Build history of the part. All positions in model axes, mm. Face numbers are marked on the shaded views. A direction names the side the tool comes from. Round coordinates to 2 decimals unless told otherwise and drop trailing zeros. Write each loop counter-clockwise with the first axis right and the second up, starting at its lowest first coordinate (ties: lowest second). Pieces come first, ordered by that corner, then holes. Notation, with made-up numbers: (45.25, 75) - (52.25, 75) arc R24 ccw to (52.25, 89) - close; hole circle Ø10 at (70, 66.25). An arc over 180 degrees is marked (long way). Answer as a JSON object with one key per item and string values. Group by question number.
Item 1: Two-plate mould, pull along Y, no slides. Class the marked faces 4, 5 and 6: +Y half, -Y half, draft (parallel to the pull), parting line (faces both ways), or undercut.
Item 2: Which spindle directions (+Z, -Z, +X, -X, +Y, -Y) get a long thin tool onto all of the face, cutting with end or side? Do the marked faces 1, 2 and 3. Say none if no direction does.
Item 3: Slice it at A-A, the plane x = 0. List the corners of the cut face in (y, z).
Item 4: Probe line 1 (Y direction, x = -15.5, z = 30.25); line 2 (X direction, y = -15.5, z = 0.7); line 3 (Y direction, x = 0, z = 33.45). List the from-to ranges inside material, lowest first. Write a range as from..to.
Item 5: Slice it at B-B, the plane z = 4. List the corners of the cut face in (x, y).
Item 6: Flat gauge pins, fed straight in: pin 1 (1.5 mm diameter, centred on y = 14, z = 35, fed in from -X); pin 2 (2 mm diameter, centred on x = -16.5, y = -11, fed in from +Z); pin 3 (0.9 mm diameter, centred on x = -16, y = -15.5, fed in from +Z); pin 4 (5 mm diameter, centred on x = 15.5, y = 15.5, fed in from -Z). Where does each tip first touch, or does it go through?
Item 7: Slice it at D-D, the plane z = 20. List the corners of the cut face in (x, y).
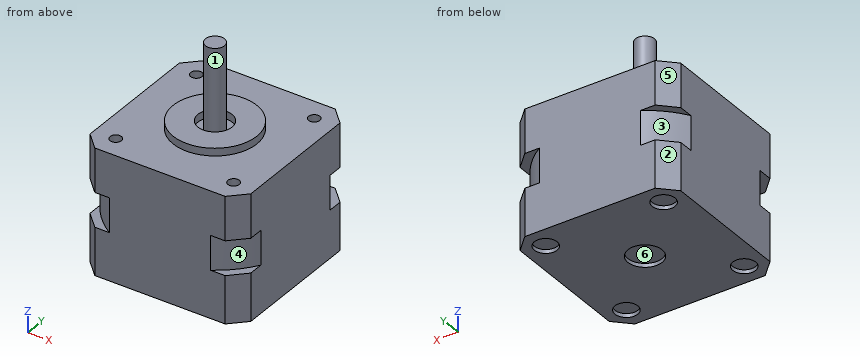
from build123d import *

# Parameters (mm, degrees)
F0_W      = 42.3
F0_H      = 42.3
F1_DEPTH  = 33
F2_SIZE   = 4
F3_R      = 11
F3_R_2    = 4.5
F4_DEPTH  = 2
F5_R      = 1.5
F6_DEPTH  = 9
F7_R      = 4.5
F7_R_2    = 3
F8_DEPTH  = 1
F9_R      = 2.5
F10_DEPTH = 22.3
F11_W     = 6.266167
F11_H     = 9


with BuildPart() as f1:
    # F0 (on Top) → F1 (new body)
    with BuildSketch(Plane.XY):
        Rectangle(F0_W, F0_H)
    extrude(amount=F1_DEPTH)

    # F2
    f2_edges = [f1.edges().sort_by_distance(p)[0] for p in [
        (21.15, -21.15, 16.5),
        (-21.15, -21.15, 16.5),
        (21.15, 21.15, 16.5),
        (-21.15, 21.15, 16.5),
    ]]
    chamfer(f2_edges, length=F2_SIZE)

    # F3 (on face) → F4 (join)
    with BuildSketch(Plane.XY.offset(33)):
        Circle(F3_R)
        Circle(F3_R_2, mode=Mode.SUBTRACT)
    extrude(amount=F4_DEPTH)

    # F5 (on face) → F6 (cut)
    with BuildSketch(Plane.XY.offset(33)):
        with Locations((15.5, 15.5)):
            Circle(F5_R)
        with Locations((15.5, -15.5)):
            Circle(F5_R)
        with Locations((-15.5, -15.5)):
            Circle(F5_R)
        with Locations((-15.5, 15.5)):
            Circle(F5_R)
    extrude(amount=-F6_DEPTH, mode=Mode.SUBTRACT)

    # F7 (on face) → F8 (cut)
    with BuildSketch(Plane(origin=(0, 0, 0), x_dir=(1, 0, 0), z_dir=(0, 0, -1))):
        Circle(F7_R)
        with Locations((-15.5, 15.5)):
            Circle(F7_R_2)
        with Locations((-15.5, -15.5)):
            Circle(F7_R_2)
        with Locations((15.5, -15.5)):
            Circle(F7_R_2)
        with Locations((15.5, 15.5)):
            Circle(F7_R_2)
    extrude(amount=-F8_DEPTH, mode=Mode.SUBTRACT)

    # F9 (on face) → F10 (join)
    with BuildSketch(Plane.XY.offset(33)):
        Circle(F9_R)
    extrude(amount=F10_DEPTH)

    # F11 (on Right) → F12 (revolve, cut)
    with BuildSketch(Plane.YZ):
        with Locations((28.133083, 17)):
            Rectangle(F11_W, F11_H)
    revolve(axis=Axis((0, 0, 12.553133), (0, 0, 1)), mode=Mode.SUBTRACT)


solid = f1.part
Geometry says:
{
 "1": {"face 4": "-Y half", "face 5": "+Y half", "face 6": "undercut"},
 "2": {"face 1": "+Z", "face 2": "+Z, -Z, -X, +Y", "face 3": "-X, +Y"},
 "3": {"outline": "(-21.15, 0) - (-4.5, 0) - (-4.5, 1) - (4.5, 1) - (4.5, 0) - (21.15, 0) - (21.15, 33) - (11, 33) - (11, 35) - (4.5, 35) - (4.5, 33) - (2.5, 33) - (2.5, 55.3) - (-2.5, 55.3) - (-2.5, 33) - (-4.5, 33) - (-4.5, 35) - (-11, 35) - (-11, 33) - (-21.15, 33) - close"},
 "4": {"line 1": "y = -21.15..-17, -14..14, 17..21.15", "line 2": "x = -21.15..-18.5, -12.5..12.5, 18.5..21.15", "line 3": "y = -11..-4.5, -2.5..2.5, 4.5..11"},
 "5": {"outline": "(-21.15, -17.15) - (-17.15, -21.15) - (17.15, -21.15) - (21.15, -17.15) - (21.15, 17.15) - (17.15, 21.15) - (-17.15, 21.15) - (-21.15, 17.15) - close"},
 "6": {"pin 1": "passes through", "pin 2": "stops at z = 33", "pin 3": "stops at z = 24", "pin 4": "stops at z = 1"},
 "7": {"outline": "(-21.15, -13.33) arc R25 ccw to (-13.33, -21.15) - (13.33, -21.15) arc R25 ccw to (21.15, -13.33) - (21.15, 13.33) arc R25 ccw to (13.33, 21.15) - (-13.33, 21.15) arc R25 ccw to (-21.15, 13.33) - close"}
}
